Answer from the drawing. Dimensions are ordinates in mm from the lowest x, y and z of the part. A direction names the side the tool comes from. Give positions to 0.01 mm unless a question says otherwise; leave off trailing zeros. Write each loop counter-clockwise with the first axis right and the second up, starting at its lowest first coordinate (ties: lowest second). Pieces come first, ordered by that corner, then holes. Notation, with made-up numbers: M 44,12 L 80,12 A26 cw 80,44 Z; hole C 63.25,44.5 d2. An arc over 180 degrees is marked long. Put each result on its own line as item: value.
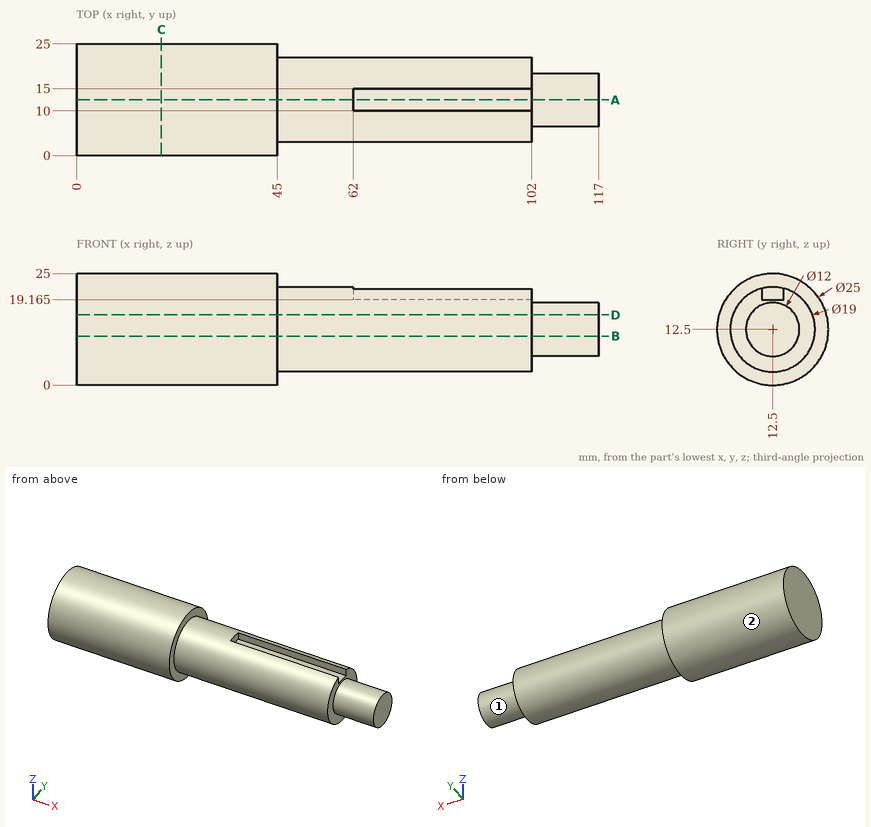
(1) Which of the six approach directions +Z, -Z, +X, -X, +Y, -Y give full straight-line access (tool end or side, diameter ignored) to the marked faces 1 and 2?
Result:
face 1: +X
face 2: +X, -X
(2) Section C-C on x = 19 is taken. Determine the outline of the cut face in (y, z).
Result:
outline: C 12.5,12.5 d25
(3) Section D-D on z = 15.75 is taken. Determine the outline of the cut face in (x, y).
Result:
outline: M 0,0.43 L 45,0.43 L 45,3.57 L 102,3.57 L 102,7.46 L 117,7.46 L 117,17.54 L 102,17.54 L 102,21.43 L 45,21.43 L 45,24.57 L 0,24.57 Z
(4) Section A-A on y = 12.5 is taken. Determine the outline of the cut face in (x, z) (3 decimals).
Result:
outline: M 0,0 L 45,0 L 45,3 L 102,3 L 102,6.5 L 117,6.5 L 117,18.5 L 102,18.5 L 102,19.165 L 62,19.165 L 62,22 L 45,22 L 45,25 L 0,25 Z
(5) Straight lines are drawn through the part: line 1 along X through (y, z) = (9, 23.75); line 2 along X through (y, z) = (12.5, 21.25); line 3 along Y through (x, z) = (35, 12.25). For each, find the intervals that lie inside material, in ascending order. Write a range as from..to.
Result:
line 1: x = 0..45
line 2: x = 0..62
line 3: y = 0..25
(6) Section B-B on z = 11 is taken. Determine the outline of the cut face in (x, y), and give its area (3 significant figures).
Result:
outline: M 0,0.09 L 45,0.09 L 45,3.12 L 102,3.12 L 102,6.69 L 117,6.69 L 117,18.31 L 102,18.31 L 102,21.88 L 45,21.88 L 45,24.91 L 0,24.91 Z
area: 2,360 mm²
(7) Given pin 1 Ø1 at (x, z) = (26, 9) entering from -Y; pin 2 Ø10 at (x, z) = (85, 4.5) entering from +Y; pin 3 Ø1.3 at (x, z) = (74, 20) entering from +Y, each flat-ended and moving along its own axis, determine where each tip first touches the part or whether it passes through.
Result:
pin 1: stops at y = 0.37
pin 2: stops at y = 21.51
pin 3: stops at y = 19.08
